Geometry: final body of the model. Coordinates: model frame, mm. A direction names the side the tool comes from. Coordinates: 2 decimals unless noted, no trailing zeros. Loops run counter-clockwise (first coordinate to the right, second up) from the corner with the lowest first, then second, coordinate; pieces in that order, holes last. Notation, with made-up numbers: (22.5, 17.5) - (30.5, 17.5) arc R20 cw to (30.5, 26.5) - close; hole circle Ø2 at (-35.75, -31). An arc over 180 degrees is marked (long way). Write each question's results on one line, items separated by ' | '. Start each with the question number.
from build123d import *

# Parameters (mm, degrees)
SKETCH2_W           = 80
SKETCH2_H           = 100
BOSS_EXTRUDE1_DEPTH = 10
SKETCH3_W           = 20
SKETCH3_H           = 100
BOSS_EXTRUDE2_DEPTH = 120
SKETCH5_R           = 2.555
CUT_EXTRUDE2_DEPTH  = 55
FILLET2_R           = 20
SKETCH4_R           = 0.75
CUT_EXTRUDE3_DEPTH  = 51


with BuildPart() as part:
    # Sketch2 → Boss-Extrude1 (new body)
    with BuildSketch(Plane(origin=(0, 0, 0), x_dir=(1, 0, 0), z_dir=(0, 1, 0))):
        Rectangle(SKETCH2_W, SKETCH2_H)
    extrude(amount=BOSS_EXTRUDE1_DEPTH)

    # Sketch3 → Boss-Extrude2 (add)
    with BuildSketch(Plane(origin=(0, 10, 0), x_dir=(1, 0, 0), z_dir=(0, 1, 0))):
        Rectangle(SKETCH3_W, SKETCH3_H)
    extrude(amount=BOSS_EXTRUDE2_DEPTH)

    # Sketch5 → Cut-Extrude2 (cut)
    with BuildSketch(Plane.XZ):
        with Locations((-25.4, -38.1)):
            Circle(SKETCH5_R)
        with Locations((25.4, -38.1)):
            Circle(SKETCH5_R)
        with Locations((-25.4, 38.1)):
            Circle(SKETCH5_R)
        with Locations((25.4, 38.1)):
            Circle(SKETCH5_R)
    extrude(amount=-CUT_EXTRUDE2_DEPTH, mode=Mode.SUBTRACT)

    # Fillet2
    fillet2_edges = [part.edges().sort_by_distance(p)[0] for p in [
        (0, 130, -50),
        (0, 130, 50),
    ]]
    fillet(fillet2_edges, radius=FILLET2_R)

    # Sketch4 → Cut-Extrude3 (cut, through all)
    with BuildSketch(Plane.ZY.offset(10)):
        with Locations((-8.5, 106.75)):
            Circle(SKETCH4_R)
        with Locations((-8.5, 90.25)):
            Circle(SKETCH4_R)
        with Locations((8.5, 90.25)):
            Circle(SKETCH4_R)
        with Locations((8.5, 106.75)):
            Circle(SKETCH4_R)
    extrude(amount=-CUT_EXTRUDE3_DEPTH, mode=Mode.SUBTRACT)


solid = part.part
1) Section query D-D on y = 76. Output: boundary loops of the cut face in (x, z), and give its area (3 significant figures).
2) Section query B-B on z = 38.1. Output: boundary loops of the cut face in (x, y) (3 decimals).
3) Section query A-A on x = 25.4. Output: boundary loops of the cut face in (y, z) (3 decimals).
4) Section query C-C on z = 21. Output: boundary loops of the cut face in (x, y), and give its area (3 significant figures).
5) Material intervals for line 1 (X direction, y = 2, z = -38); line 2 (Z direction, x = 1, y = 106.75); line 3 (Z direction, x = 25, y = 7), sorted ascending. Write a range as [from, to].
6) Pin query (flat end, axial travel): pin 1 Ø5 at (x, z) = (-21, 29) entering from +Y; pin 2 Ø0.9 at (y, z) = (106.75, 8.5) entering from +X; pin 3 Ø1.7 at (y, z) = (106.75, -8.5) entering from -X; pin 4 Ø4 at (y, z) = (51, -5.5) entering from +X. Return the tip coordinate at first contact, or that it passes through.
7) Access query for faces 1 (the cylindrical face through (0.14, 123.986, -44.297)), 2 (the flat face through (-25, 10, -1)), 3 (the flat face through (10, 69, 1)). Directions: +Z, -Z, +X, -X, +Y, -Y. A direction counts if a zero-diameter tool reaches every point of the face in a straight line with its end or side. Return the directions, or none.
8) Pull-direction query (X, two-part tool) for faces 4 (the flat face through (-40, 5, 1)), 5 (the flat face through (25, 10, -1)), 6 (the cylindrical face through (-27.43, 4.93, 36.55)); classes: released by +X, released by -X, zero draft, split by the parting line, or undercut.
Returned:
1) outline: (-10, -50) - (10, -50) - (10, 50) - (-10, 50) - close | area: 2,000 mm²
2) outline: (-40, 0) - (-27.955, 0) - (-27.955, 10) - (-40, 10) - close; (-22.845, 0) - (22.845, 0) - (22.845, 10) - (10, 10) - (10, 128.286) - (-10, 128.286) - (-10, 10) - (-22.845, 10) - close; (27.955, 0) - (40, 0) - (40, 10) - (27.955, 10) - close
3) outline: (0, -50) - (10, -50) - (10, -40.655) - (0, -40.655) - close; (0, -35.545) - (10, -35.545) - (10, 35.545) - (0, 35.545) - close; (0, 40.655) - (10, 40.655) - (10, 50) - (0, 50) - close
4) outline: (-40, 0) - (40, 0) - (40, 10) - (10, 10) - (10, 130) - (-10, 130) - (-10, 10) - (-40, 10) - close | area: 3,200 mm²
5) line 1: x = [-40, -27.95], [-22.85, 22.85], [27.95, 40] | line 2: z = [-50, -9.25], [-7.75, 7.75], [9.25, 50] | line 3: z = [-50, -40.62], [-35.58, 35.58], [40.62, 50]
6) pin 1: stops at y = 10 | pin 2: passes through | pin 3: stops at x = -10 | pin 4: stops at x = 10
7) face 1: -Z, +X, -X, +Y | face 2: +Z, -Z, -X, +Y | face 3: +Z, -Z, +X, +Y
8) face 4: released by -X | face 5: zero draft | face 6: undercut
